from build123d import *

# Parameters (mm, degrees)
F0_R     = 5
F1_DEPTH = 19.05


with BuildPart() as f1:
    # F0 (on Top) → F1 (new body)
    with BuildSketch(Plane.XY):
        with BuildLine():
            Line((-50.8, -50.8), (50.8, -50.8))
            Line((50.8, -50.8), (127, -50.8))
            Line((127, -50.8), (127, -38.1))
            Line((127, -38.1), (127, 38.1))
            Line((127, 38.1), (63.5, 38.1))
            ThreePointArc((63.5, 38.1), (54.519744, 41.819744), (50.8, 50.8))
            Line((50.8, 50.8), (50.8, 69.85))
            Line((50.8, 69.85), (-50.8, 69.85))
            Line((-50.8, 69.85), (-50.8, 50.8))
            ThreePointArc((-50.8, 50.8), (-54.519744, 41.819744), (-63.5, 38.1))
            Line((-63.5, 38.1), (-127, 38.1))
            Line((-127, 38.1), (-127, -38.1))
            Line((-127, -38.1), (-127, -50.8))
            Line((-127, -50.8), (-50.8, -50.8))
        make_face()
        with BuildLine():
            ThreePointArc((-86.57349, -41.11626), (-84.19224, -38.73501), (-81.81099, -41.11626))
            ThreePointArc((-81.81099, -41.11626), (-84.19224, -43.49751), (-86.57349, -41.11626))
        make_face(mode=Mode.SUBTRACT)
        with BuildLine():
            ThreePointArc((-31.70949, -41.11626), (-29.32824, -38.73501), (-26.94699, -41.11626))
            ThreePointArc((-26.94699, -41.11626), (-29.32824, -43.49751), (-31.70949, -41.11626))
        make_face(mode=Mode.SUBTRACT)
        with BuildLine():
            ThreePointArc((12.699988, -6.35), (25.399988, -19.05), (12.699988, -31.75))
            Line((12.699988, -31.75), (-6.350012, -31.75))
            ThreePointArc((-6.350012, -31.75), (-10.840141, -29.890128), (-12.700012, -25.4))
            Line((-12.700012, -25.4), (-12.700012, 6.35))
            ThreePointArc((-12.700012, 6.35), (-25.400012, 19.05), (-12.700012, 31.75))
            Line((-12.700012, 31.75), (6.349988, 31.75))
            ThreePointArc((6.349988, 31.75), (10.840116, 29.890128), (12.699988, 25.4))
            Line((12.699988, 25.4), (12.699988, -6.35))
        make_face(mode=Mode.SUBTRACT)
        with BuildLine():
            ThreePointArc((31.79051, -41.11626), (34.17176, -38.73501), (36.55301, -41.11626))
            ThreePointArc((36.55301, -41.11626), (34.17176, -43.49751), (31.79051, -41.11626))
        make_face(mode=Mode.SUBTRACT)
        with BuildLine():
            ThreePointArc((87.35301, -41.11626), (84.97176, -43.49751), (82.59051, -41.11626))
            ThreePointArc((82.59051, -41.11626), (84.97176, -38.73501), (87.35301, -41.11626))
        make_face(mode=Mode.SUBTRACT)
        with Locations((-33.655, 52.705)):
            Circle(F0_R, mode=Mode.SUBTRACT)
        with Locations((-16.51, 52.705)):
            Circle(F0_R, mode=Mode.SUBTRACT)
        with Locations((16.51, 52.705)):
            Circle(F0_R, mode=Mode.SUBTRACT)
        with Locations((33.655, 52.705)):
            Circle(F0_R, mode=Mode.SUBTRACT)
    extrude(amount=-F1_DEPTH)


with BuildPart() as f2_1:
    # F2: copy of F1
    add(f1.part)


with BuildPart() as f4_1:
    # F4: copy of F1
    add(f1.part)


solid = f1.part
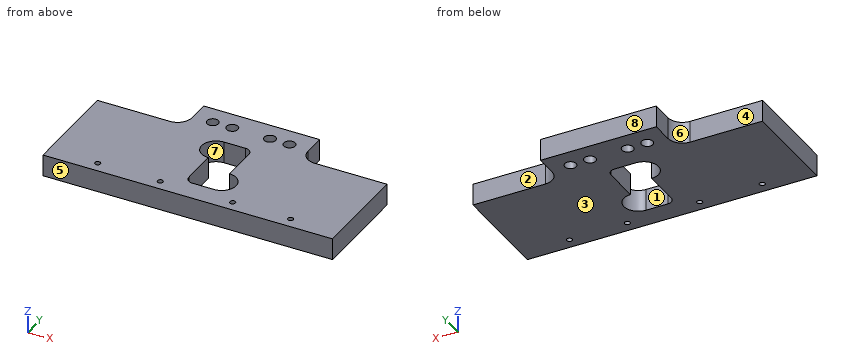
Can you work these out from the model? Positions are in its coordinate system, mm. Face numbers are marked on the shaded views. A direction names the side the tool comes from. Coordinates: 2 decimals unless noted, no trailing zeros. Write each loop counter-clockwise with the first axis right and the second up, starting at its lowest first coordinate (ties: lowest second). Pieces come first, ordered by that corner, then holes. Notation, with made-up numbers: (13, -38) -> (55, -38) arc R22 cw to (55, -32) -> close; hole circle Ø2 at (48, 75). An arc over 180 degrees is marked (long way). Write item = value, one per line.
(1) If I drill on probe 1 along Y at (x, z) = (7, -17); probe 2 along Y at (x, z) = (-16.51, -14.25) (3 decimals); probe 3 along X at (y, z) = (65.5, -16), over which ranges is the centre line in solid material (lowest first)?
Verdict:
probe_1 = -50.8 to -31.75, 31.72 to 69.85
probe_2 = -50.8 to 6.935, 31.165 to 47.705, 57.705 to 69.85
probe_3 = -50.8 to 50.8
(2) Imagine slicing it at D-D (x = -92.5). Please give me the cut outline in (y, z).
Verdict:
outline = (-50.8, -19.05) -> (38.1, -19.05) -> (38.1, 0) -> (-50.8, 0) -> close
(3) Imagine slicing it at A-A (x = -0.5). Please give me the cut outline in (y, z), and give its area (3 significant figures).
Verdict:
outline = (-50.8, -19.05) -> (-31.75, -19.05) -> (-31.75, 0) -> (-50.8, 0) -> close; (31.75, -19.05) -> (69.85, -19.05) -> (69.85, 0) -> (31.75, 0) -> close
area = 1,090 mm^2
(4) For pin 1 (4 mm diameter, centred on x = 34.17, y = -41.12, fed in from -Z); pin 2 (5.5 mm diameter, centred on x = 80, z = -12, fed in from +Y); pin 3 (9.5 mm diameter, centred on y = 57.5, z = -11, fed in from -X), each with a flat end and sliding along its axis, tell me the tip position at first contact or that it passes through.
Verdict:
pin_1 = through
pin_2 = 38.1
pin_3 = -50.8
(5) On a 3-axis mill with a long thin cutter (end or side, diameter ignored), from which of +Z, -Z, +X, -X, +Y, -Y can I reach the whole of each face in a straight line? I mean the marked faces 1, 2, 3, 4 and 5. Say none if no direction works.
Verdict:
face_1 = +Z, -Z
face_2 = +Z, -Z, +X, +Y
face_3 = -Z, +X, -X, +Y, -Y
face_4 = +Z, -Z, -X, +Y
face_5 = +Z, -Z, +X, -X, -Y
(6) Thinking about a two-plate mould opening in X: for the marked faces 6, 7 and 8, which applies, +X half, -X half, draft (parallel to the pull), parting line (faces both ways), or undercut?
Verdict:
face_6 = -X half
face_7 = undercut
face_8 = draft
(7) Imagine slicing it at B-B (y = -19.05). Please give me the cut outline in (x, z), and give its area (3 significant figures).
Verdict:
outline = (-127, -19.05) -> (-12.7, -19.05) -> (-12.7, 0) -> (-127, 0) -> close; (25.4, -19.05) -> (127, -19.05) -> (127, 0) -> (25.4, 0) -> close
area = 4,110 mm^2
(8) Imagine slicing it at C-C (z = -10.5). State how many separate pieces and enclosed holes the cut face has, and give its area (3 significant figures).
Verdict:
separate_pieces = 1
enclosed_holes = 9
area = 23,400 mm^2
